Verification items for the finished model (mm, model axes). A direction names the side the tool comes from. Give positions to 0.01 mm unless a question says otherwise; leave off trailing zeros. Write each loop counter-clockwise with the first axis right and the second up, starting at its lowest first coordinate (ties: lowest second). Pieces come first, ordered by that corner, then holes.
from build123d import *

# Parameters (mm, degrees)
F1_DEPTH = 15


with BuildPart() as f1:
    # F0 (on Top) → F1 (new body)
    with BuildSketch(Plane.XY):
        with BuildLine():
            Line((11.5, -2.2), (8.951817, -2.2))
            Line((8.951817, -2.2), (8.951817, -2.5))
            Line((8.951817, -2.5), (3.380814, -2.5))
            ThreePointArc((3.380814, -2.5), (3.139489, -2.790809), (3, -3.142021))
            ThreePointArc((3, -3.142021), (2.434954, -4.046773), (1.428434, -4.4))
            Line((1.428434, -4.4), (0, -4.4))
            Line((0, -4.4), (-1.428434, -4.4))
            ThreePointArc((-1.428434, -4.4), (-2.434954, -4.046773), (-3, -3.142021))
            ThreePointArc((-3, -3.142021), (-3.139489, -2.790809), (-3.380814, -2.5))
            Line((-3.380814, -2.5), (-8.951817, -2.5))
            Line((-8.951817, -2.5), (-8.951817, -2.2))
            Line((-8.951817, -2.2), (-11.5, -2.2))
            ThreePointArc((-11.5, -2.2), (-12.240729, -2.342227), (-12.876106, -2.748679))
            Line((-12.876106, -2.748679), (-15.143142, -4.898226))
            ThreePointArc((-15.143142, -4.898226), (-16.698226, -4.856858), (-16.656858, -3.301774))
            ThreePointArc((-16.656858, -3.301774), (-16.632203, -2.601088), (-17.332363, -2.564418))
            ThreePointArc((-17.332363, -2.564418), (-17.546933, -5.924986), (-14.187646, -6.158764))
            Line((-14.187646, -6.158764), (-13.658737, -5.70133))
            ThreePointArc((-13.658737, -5.70133), (-12.02897, -4.735894), (-10.164732, -4.4))
            Line((-10.164732, -4.4), (-4.96455, -4.4))
            ThreePointArc((-4.96455, -4.4), (-4.582113, -4.49077), (-4.281257, -4.743718))
            ThreePointArc((-4.281257, -4.743718), (-3.269164, -5.594645), (-1.98263, -5.9))
            Line((-1.98263, -5.9), (0, -5.9))
            Line((0, -5.9), (1.98263, -5.9))
            ThreePointArc((1.98263, -5.9), (3.269164, -5.594645), (4.281257, -4.743718))
            ThreePointArc((4.281257, -4.743718), (4.582113, -4.49077), (4.96455, -4.4))
            Line((4.96455, -4.4), (10.164732, -4.4))
            ThreePointArc((10.164732, -4.4), (12.02897, -4.735894), (13.658737, -5.70133))
            Line((13.658737, -5.70133), (14.187646, -6.158764))
            ThreePointArc((14.187646, -6.158764), (17.546933, -5.924986), (17.332363, -2.564418))
            ThreePointArc((17.332363, -2.564418), (16.632203, -2.601088), (16.656858, -3.301774))
            ThreePointArc((16.656858, -3.301774), (16.698226, -4.856858), (15.143142, -4.898226))
            Line((15.143142, -4.898226), (12.876106, -2.748679))
            ThreePointArc((12.876106, -2.748679), (12.240729, -2.342227), (11.5, -2.2))
        make_face()
    extrude(amount=F1_DEPTH)


solid = f1.part
Item 1: Depth check by flat-ended pin: pin 1 (1.5 mm diameter, centred on y = -6, z = 8.5, fed in from -X); pin 2 (5.5 mm diameter, centred on x = 7.5, z = 9, fed in from -Y); pin 3 (5.5 mm diameter, centred on x = -6.5, z = 5.5, fed in from -Y); pin 4 (1.5 mm diameter, centred on x = -1, y = -3, fed in from +Z). Enter the tip coordinate at first touch or a pass-through.
Answer key:
pin 1: stops at x = -17.96
pin 2: stops at y = -4.43
pin 3: stops at y = -5.29
pin 4: passes through
Item 2: Sectioned sample at C-C on x = -15.9. Record the cut outline in (y, z), then the cut area to 3 significant figures.
Answer key:
outline: (-6.74, 0) - (-5.2, 0) - (-5.2, 15) - (-6.74, 15) - close
area: 23.0 mm2
Item 3: Sectioned sample at B-B on x = -0.5. Record the cut outline in (y, z).
Answer key:
outline: (-5.9, 0) - (-4.4, 0) - (-4.4, 15) - (-5.9, 15) - close
Item 4: Release check for a two-part mould opening along Y. For faces 4 (the face through (-16.681, -4.874, 7.395)), 5 (the face through (12.251, -2.346, 7.395)), 6 (the face through (12.004, -4.727, 7.395)), 7 (the face through (16.64, -2.59, 7.4)) record: released by +Y, released by -Y, zero draft, split by the parting line, or undercut.
Answer key:
face 4: undercut
face 5: released by +Y
face 6: released by -Y
face 7: undercut
Item 5: Set-up check for faces 1 (the face through (-12.23, -2.34, 7.4)), 2 (the face through (0, -5.9, 7)), 3 (the face through (16.715, -4.839, 7.395)): record each of +Z, -Z, +X, -X, +Y, -Y from which the full face is reachable in a straight line by a thin tool's end or side.
Answer key:
face 1: +Z, -Z, +Y
face 2: +Z, -Z, -Y
face 3: +Z, -Z
Item 6: Scan lines: line 1 along X through (y, z) = (-5.5, 7.75); line 2 along X through (y, z) = (-4.9, 1.75); line 3 along Y through (x, z) = (5, 10). Record each from-to range of solid material in increasing order.
Answer key:
line 1: x = -17.84 to -13.41, -3.44 to 3.44, 13.41 to 17.84
line 2: x = -18.07 to -16.65, -15.15 to -12.42, -4.16 to 4.16, 12.42 to 15.15, 16.65 to 18.07
line 3: y = -4.4 to -2.5
